Answer from the drawing. Dimensions are ordinates in mm from the lowest x, y and z of the part. A direction names the side the tool comes from. Coordinates: 2 decimals unless noted, no trailing zeros. Write each loop counter-clockwise with the first axis right and the second up, starting at its lowest first coordinate (ties: lowest second). Pieces come first, ordered by that corner, then holes. Notation, with made-up numbers: (19.5, 23.25) -> (53.5, 23.25) arc R27 ccw to (53.5, 47.25) -> close; hole circle Ø3 at (60, 52). An arc over 180 degrees is marked (long way). Answer as a JSON object with one key per item and string values. Group by question number.
(1) Find section A-A (x = 43.5). Give the vertices of the cut face in (y, z), then the cut area to 3 significant figures.
(2) A straight line is drawn through the part: L1, parallel to X at y = 116, z = 15.5. Find the intervals that lie inside material, in ascending order.
(3) For a pull along X with two mould halves and no side action, classify the marked faces 1, 2 and 3 as +X half, -X half, draft (parallel to the pull), parting line (faces both ways), or undercut.
(4) Which of the six approach directions +Z, -Z, +X, -X, +Y, -Y give full straight-line access (tool end or side, diameter ignored) to the marked faces 4 and 5?
(5) Find section C-C (z = 12). Give the vertices of the cut face in (x, y) (3 decimals).
(6) A flat-ended cylindrical pin translates along its axis: P1, Ø3.5, axis at x = 9.525, y = 187.325, coming from the -Z side. Find the tip coordinate at first contact, or state that the pin passes through.
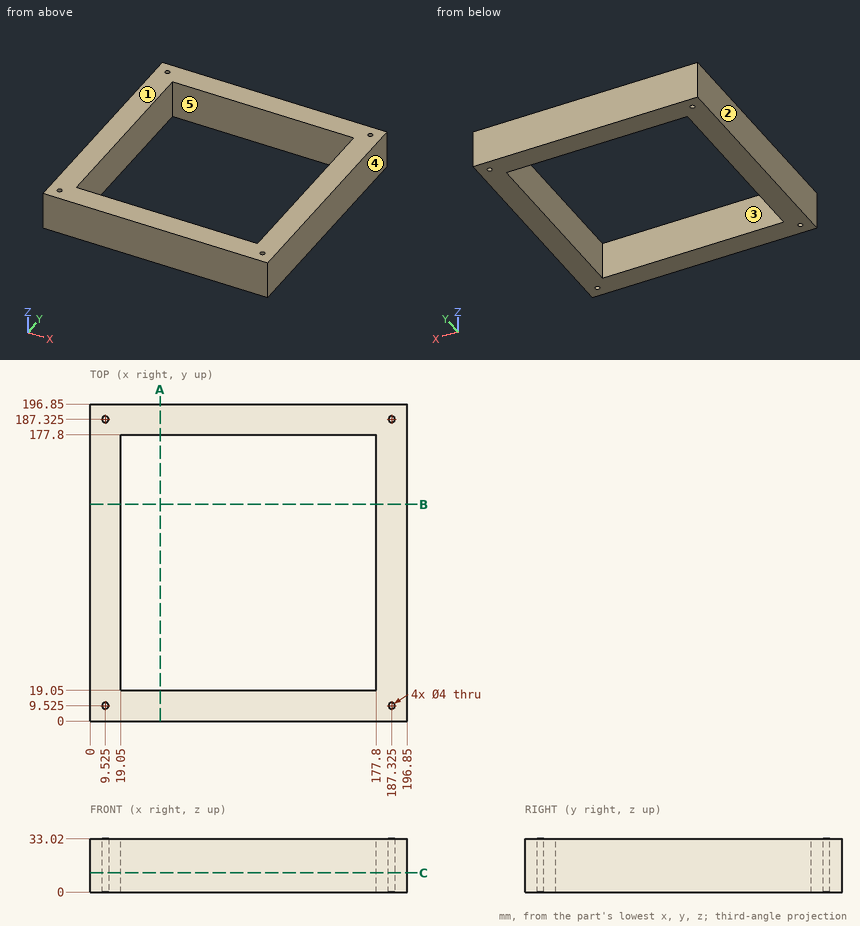
Results below:
{
 "1": {"outline": "(0, 0) -> (19.05, 0) -> (19.05, 33.02) -> (0, 33.02) -> close; (177.8, 0) -> (196.85, 0) -> (196.85, 33.02) -> (177.8, 33.02) -> close", "area": "1,260 mm2"},
 "2": {"L1": "x = 0 to 19.05, 177.8 to 196.85"},
 "3": {"face 1": "draft", "face 2": "-X half", "face 3": "undercut"},
 "4": {"face 4": "+Z, -Z, +X, +Y, -Y", "face 5": "+Z, -Z"},
 "5": {"outline": "(0, 0) -> (196.85, 0) -> (196.85, 196.85) -> (0, 196.85) -> close; hole circle Ø4 at (9.525, 9.525); hole circle Ø4 at (9.525, 187.325); hole (19.05, 19.05) -> (177.8, 19.05) -> (177.8, 177.8) -> (19.05, 177.8) -> close; hole circle Ø4 at (187.325, 9.525); hole circle Ø4 at (187.325, 187.325)"},
 "6": {"P1": "passes through"}
}
